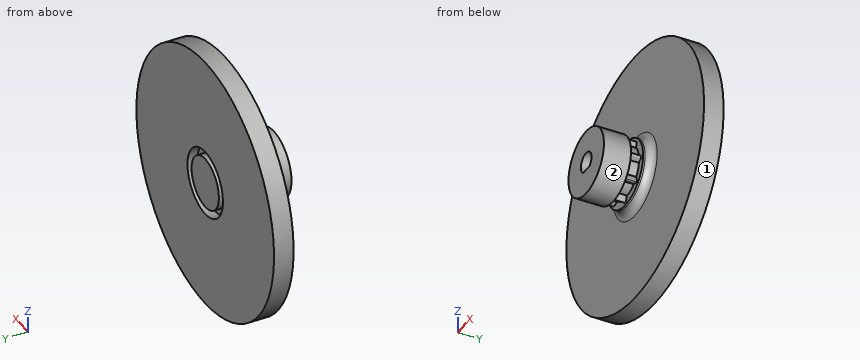
from build123d import *

# Parameters (mm, degrees)
BOSS_EXTRUDE1_DEPTH      = 2.5
BOSS_EXTRUDE1_DEPTH_BACK = 2.5
SKETCH1_R                = 33
SKETCH1_R_2              = 8.5
BOSS_EXTRUDE2_DEPTH      = 2.5
BOSS_EXTRUDE3_DEPTH      = 2.5
BOSS_EXTRUDE3_DEPTH_BACK = 15
SKETCH1_5_R              = 6.55
SKETCH1_6_R              = 8.5
SKETCH1_6_R_2            = 6.55
BOSS_EXTRUDE4_DEPTH      = 5
BOSS_EXTRUDE5_START      = -6.9
SKETCH2_R                = 8.5
SKETCH2_R_2              = 2.55
BOSS_EXTRUDE5_DEPTH      = 6.9
FILLET1_R                = 2
BOSS_EXTRUDE6_DEPTH      = 3.01


with BuildPart() as part:
    # Sketch1 → Boss-Extrude1 (new, two sides: drawn at the far end of the back side and taken through both)
    with BuildSketch(Plane(origin=(0, 0, 0), x_dir=(1, 0, 0), z_dir=(0, 1, 0)).offset(-BOSS_EXTRUDE1_DEPTH_BACK)):
        with Locations(Location((0, 0, 0), (0, 0, 270))):
            Circle(SKETCH1_R)
        with Locations(Location((0, 0, 0), (0, 0, 270))):
            Circle(SKETCH1_R_2, mode=Mode.SUBTRACT)
    extrude(amount=BOSS_EXTRUDE1_DEPTH + BOSS_EXTRUDE1_DEPTH_BACK)



with BuildPart() as body_2:
    # Sketch1<4> → Boss-Extrude2 (new body)
    with BuildSketch(Plane(origin=(0, 0, 0), x_dir=(1, 0, 0), z_dir=(0, 1, 0))):
        with BuildLine():
            ThreePointArc((-1.53, 2.04), (-2.41914241, -0.806380803), (0, -2.55))
            Line((0, -2.55), (0, 2.04))
            Line((0, 2.04), (-1.53, 2.04))
        make_face()
        with BuildLine():
            Line((0, 2.04), (0, -2.55))
            ThreePointArc((0, -2.55), (1.803122292, -1.803122292), (2.55, 0))
            ThreePointArc((2.55, 0), (2.280789337, 1.140394669), (1.53, 2.04))
            Line((1.53, 2.04), (0, 2.04))
        make_face()
    extrude(amount=BOSS_EXTRUDE2_DEPTH)

    # Sketch1<5> → Boss-Extrude3 (add, two sides: drawn at the far end of the back side and taken through both)
    with BuildSketch(Plane(origin=(0, 0, 0), x_dir=(1, 0, 0), z_dir=(0, 1, 0)).offset(-BOSS_EXTRUDE3_DEPTH_BACK)):
        with Locations(Location((0, 0, 0), (0, 0, 270))):
            Circle(SKETCH1_5_R)
        with BuildLine():
            Line((-1.53, 2.04), (1.53, 2.04))
            ThreePointArc((1.53, 2.04), (0, -2.55), (-1.53, 2.04))
        make_face(mode=Mode.SUBTRACT)
    extrude(amount=BOSS_EXTRUDE3_DEPTH + BOSS_EXTRUDE3_DEPTH_BACK)


with BuildPart() as part_1:
    add(part.part)

    add(body_2.part)  # Boss-Extrude4 merges body 2
    # Sketch1<6> → Boss-Extrude4 (add)
    with BuildSketch(Plane(origin=(0, 0, 0), x_dir=(1, 0, 0), z_dir=(0, 1, 0))):
        with Locations(Location((0, 0, 0), (0, 0, 270))):
            Circle(SKETCH1_6_R)
        with Locations(Location((0, 0, 0), (0, 0, 270))):
            Circle(SKETCH1_6_R_2, mode=Mode.SUBTRACT)
    extrude(amount=-BOSS_EXTRUDE4_DEPTH)

    # Sketch2 → Boss-Extrude5 (add)
    with BuildSketch(Plane(origin=(0, -8.1, 0), x_dir=(1, 0, 0), z_dir=(0, 1, 0)).offset(BOSS_EXTRUDE5_START)):
        with Locations(Location((0, 0, 0), (0, 0, 270))):
            Circle(SKETCH2_R)
        Circle(SKETCH2_R_2, mode=Mode.SUBTRACT)
    extrude(amount=BOSS_EXTRUDE5_DEPTH)

    # Fillet1
    fillet1_edges = [part_1.edges().sort_by_distance(p)[0] for p in [
        (0, -2.5, -8.5),
    ]]
    fillet(fillet1_edges, radius=FILLET1_R)

    # Sketch3 → Boss-Extrude6 (add)
    with BuildSketch(Plane(origin=(0, -8.1, 0), x_dir=(1, 0, 0), z_dir=(0, 1, 0))):
        with BuildLine():
            ThreePointArc((6.489574687, 0.887648796), (6.55, 0), (6.489574687, -0.887648796))
            add(Edge.make_bspline(
                [(6.489574687, -0.887648796), (7.8, -0.48452531), (7.8, 0)],
                knots=[5.695086191, 5.695086191, 5.695086191, 6.283185307, 6.283185307, 6.283185307], degree=2, weights=[1, 0.957078041, 1]))
            add(Edge.make_bspline(
                [(7.8, 0), (7.8, 0.48452531), (6.489574687, 0.887648796)],
                knots=[0, 0, 0, 0.588099116, 0.588099116, 0.588099116], degree=2, weights=[1, 0.957078041, 1]))
        make_face()
        with BuildLine():
            ThreePointArc((3.961159785, 5.216484751), (4.631549417, 4.631549417), (5.216484751, 3.961159785))
            add(Edge.make_bspline(
                [(5.216484751, 3.961159785), (5.858044026, 5.172821761), (5.515432893, 5.515432893)],
                knots=[5.695086191, 5.695086191, 5.695086191, 6.283185307, 6.283185307, 6.283185307], degree=2, weights=[1, 0.957078041, 1]))
            add(Edge.make_bspline(
                [(5.515432893, 5.515432893), (5.172821761, 5.858044026), (3.961159785, 5.216484751)],
                knots=[0, 0, 0, 0.588099116, 0.588099116, 0.588099116], degree=2, weights=[1, 0.957078041, 1]))
        make_face()
        with BuildLine():
            add(Edge.make_bspline(
                [(3.972298874, -5.208007456), (6.522331769, -6.529808173), (5.201644202, -3.98062779)],
                knots=[2.567584119, 2.567584119, 2.567584119, 3.715272936, 3.715272936, 3.715272936], degree=2, weights=[1, 0.839820193, 1]))
            ThreePointArc((5.201644202, -3.98062779), (4.627842164, -4.635253704), (3.972298874, -5.208007456))
        make_face()
        with BuildLine():
            ThreePointArc((-0.911324659, 6.486292267), (-0.00524075, 6.549997903), (0.900943942, 6.487742289))
            add(Edge.make_bspline(
                [(0.900943942, 6.487742289), (0.491618387, 7.85844559), (-0.004973928, 7.85844559)],
                knots=[5.681298558, 5.681298558, 5.681298558, 6.283185307, 6.283185307, 6.283185307], degree=2, weights=[1, 0.955057278, 1]))
            add(Edge.make_bspline(
                [(-0.004973928, 7.85844559), (-0.501854156, 7.85844559), (-0.911324659, 6.486292267)],
                knots=[0, 0, 0, 0.602215002, 0.602215002, 0.602215002], degree=2, weights=[1, 0.955008614, 1]))
        make_face()
        with BuildLine():
            add(Edge.make_bspline(
                [(-0.873777918, -6.491456859), (-0.005286616, -9.229256662), (0.863388985, -6.492846792)],
                knots=[2.567584119, 2.567584119, 2.567584119, 3.715272936, 3.715272936, 3.715272936], degree=2, weights=[1, 0.839820193, 1]))
            ThreePointArc((0.863388985, -6.492846792), (-0.00524075, -6.549997903), (-0.873777918, -6.491456859))
        make_face()
        with BuildLine():
            ThreePointArc((-5.230905092, 3.9420974), (-4.635253704, 4.627842164), (-3.950462996, 5.224590138))
            add(Edge.make_bspline(
                [(-3.950462996, 5.224590138), (-5.209133471, 5.904386861), (-5.560277264, 5.553243068)],
                knots=[5.681298558, 5.681298558, 5.681298558, 6.283185307, 6.283185307, 6.283185307], degree=2, weights=[1, 0.955057278, 1]))
            add(Edge.make_bspline(
                [(-5.560277264, 5.553243068), (-5.911624643, 5.201895689), (-5.230905092, 3.9420974)],
                knots=[0, 0, 0, 0.602215002, 0.602215002, 0.602215002], degree=2, weights=[1, 0.955008614, 1]))
        make_face()
        with BuildLine():
            add(Edge.make_bspline(
                [(-5.216484751, -3.961159785), (-6.629151931, -6.629151931), (-3.961159785, -5.216484751)],
                knots=[2.553493537, 2.553493537, 2.553493537, 3.72969177, 3.72969177, 3.72969177], degree=2, weights=[1, 0.831996755, 1]))
            ThreePointArc((-3.961159785, -5.216484751), (-4.631549417, -4.631549417), (-5.216484751, -3.961159785))
        make_face()
        with BuildLine():
            ThreePointArc((-6.489574687, -0.887648796), (-6.55, 0), (-6.489574687, 0.887648796))
            add(Edge.make_bspline(
                [(-6.489574687, 0.887648796), (-9.375036568, 0), (-6.489574687, -0.887648796)],
                knots=[2.553493537, 2.553493537, 2.553493537, 3.72969177, 3.72969177, 3.72969177], degree=2, weights=[1, 0.831996755, 1]))
        make_face()
    extrude(amount=BOSS_EXTRUDE6_DEPTH)


solid = part_1.part
Could you check a few things on this model? Use its own coordinates, in mm. Face numbers are marked on the shaded views. A direction names the side the tool comes from. Give positions to 0.01 mm unless a question says otherwise; leave off trailing zeros. Order: outer loops, then holes, each group sorted by start corner. A loop starts at its lowest first (then second) coordinate and runs counter-clockwise, first axis right, second up. Notation, with made-up numbers: (-15.75, 70.5) - (12.25, 70.5) arc R10 ccw to (12.25, 87.5) - close; hole circle Ø3 at (49.5, 13). An arc over 180 degrees is marked (long way). One line per item, written item: value. Start each with the question number.
1. For P1, Ø0.9, axis at x = 0, y = -11, coming from the +Z side; P2, Ø8, axis at y = -4, z = -1, coming from the -X side; P3, Ø10, axis at y = -13, z = -7, coming from the -X side, each with a flat end and sliding along its axis, tell me the tip position at first contact or that it passes through.
2. Imagine slicing it at A-A on y = 1. List the corners of the cut face in (x, z) for me.
3. Imagine slicing it at D-D on x = 13. List the corners of the cut face in (y, z) for me.
4. If I drill on probe 1 along X at (y, z) = (0.5, 0); probe 2 along X at (y, z) = (-9.5, 0); probe 3 along X at (y, z) = (-5.5, 0), over which ranges is the centre line in solid material (lowest first)?
5. For the marked faces 1 and 2, which set-ups out of +Z, -Z, +X, -X, +Y, -Y let a thin tool reach every point of the face, with its end or its side?
6. Imagine slicing it at C-C on z = -25. List the corners of the cut face in (x, y) for me, plus the area to 3 significant figures.
7. Imagine slicing it at B-B on y = -9.75. List the corners of the cut face in (x, z) for me, plus the area to 3 significant figures.
Values:
1. P1: z = 8.5
1. P2: x = -33
1. P3: x = -8.26
2. outline: circle Ø66 at (0, 0); circle Ø13.1 at (0, 0); hole circle Ø17 at (0, 0)
3. outline: (-2.5, -30.33) - (2.5, -30.33) - (2.5, 30.33) - (-2.5, 30.33) - close
4. probe 1: -33 to -8.5, -6.55 to 6.55, 8.5 to 33
4. probe 2: -8.5 to -2.55, 2.55 to 8.5
4. probe 3: -7.8 to -2.55, 2.55 to 7.8
5. face 1: +Y, -Y
5. face 2: -Y
6. outline: (-21.54, -2.5) - (21.54, -2.5) - (21.54, 2.5) - (-21.54, 2.5) - close
6. area: 215 mm²
7. outline: circle Ø17 at (0, 0); hole (-1.53, -2.04) - (1.53, -2.04) arc R2.55 ccw (long way) to start
7. area: 208 mm²
